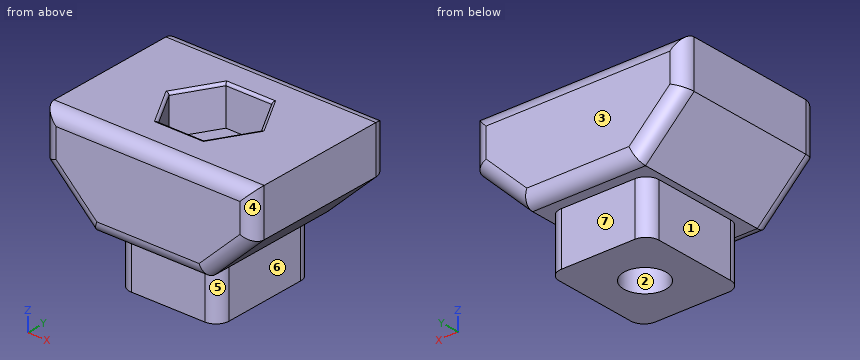
from build123d import *

# Parameters (mm, degrees)
BOSS_EXTRUDE1_DEPTH = 6
SKETCH2_W           = 7.6
SKETCH2_H           = 8.4
BOSS_EXTRUDE2_DEPTH = 4
FILLET1_R           = 1
SKETCH3_R           = 1.6
CUT_EXTRUDE1_DEPTH  = 12.2
FILLET2_R           = 1
CUT_EXTRUDE2_DEPTH  = 3
FILLET3_R           = 0.2


with BuildPart() as part:
    # Sketch1 → Boss-Extrude1 (new body, symmetric)
    with BuildSketch(Plane(origin=(0, 0, 0), x_dir=(1, 0, 0), z_dir=(0, 1, 0))):
        Polygon((-8, 0), (8, 0), (8, 3.6), (4.3, 7.2), (-4.3, 7.2), (-8, 3.6), align=None)
    extrude(amount=BOSS_EXTRUDE1_DEPTH, both=True)

    # Sketch2 → Boss-Extrude2 (add)
    with BuildSketch(Plane(origin=(0, 0, -7.2), x_dir=(-1, 0, 0), z_dir=(0, 0, -1))):
        Rectangle(SKETCH2_W, SKETCH2_H)
    extrude(amount=BOSS_EXTRUDE2_DEPTH)

    # Fillet1
    fillet1_edges = [part.edges().sort_by_distance(p)[0] for p in [
        (-6.15, 6, -5.4),
        (-8, 6, -1.8),
        (0, 6, 0),
        (8, 6, -1.8),
        (6.15, 6, -5.4),
        (8, -6, -1.8),
        (0, -6, 0),
        (-8, -6, -1.8),
        (-6.15, -6, -5.4),
        (0, -6, -7.2),
        (6.15, -6, -5.4),
        (0, 6, -7.2),
    ]]
    fillet(fillet1_edges, radius=FILLET1_R)

    # Sketch3 → Cut-Extrude1 (cut, through all)
    with BuildSketch(Plane(origin=(0, 0, -11.2), x_dir=(-1, 0, 0), z_dir=(0, 0, -1))):
        Circle(SKETCH3_R)
    extrude(amount=-CUT_EXTRUDE1_DEPTH, mode=Mode.SUBTRACT)

    # Fillet2
    fillet2_edges = [part.edges().sort_by_distance(p)[0] for p in [
        (-3.8, -4.2, -9.2),
        (-3.8, 4.2, -9.2),
        (3.8, 4.2, -9.2),
        (3.8, -4.2, -9.2),
    ]]
    fillet(fillet2_edges, radius=FILLET2_R)

    # Sketch4 → Cut-Extrude2 (cut)
    with BuildSketch(Plane.XY):
        Polygon((3.5, 0), (1.75, 3.031088913), (-1.75, 3.031088913), (-3.5, 0), (-1.75, -3.031088913), (1.75, -3.031088913), align=None)
    extrude(amount=-CUT_EXTRUDE2_DEPTH, mode=Mode.SUBTRACT)

    # Fillet3
    fillet3_edges = [part.edges().sort_by_distance(p)[0] for p in [
        (2.625, -1.515544457, 0),
        (2.625, 1.515544457, 0),
        (0, 3.031088913, 0),
        (-2.625, 1.515544457, 0),
        (-2.625, -1.515544457, 0),
        (0, -3.031088913, 0),
    ]]
    fillet(fillet3_edges, radius=FILLET3_R)


solid = part.part
Here's how the part is built. I have some questions about the finished solid (model axes, mm). Face numbers are marked on the shaded views. A direction names the side the tool comes from. Coordinates: 2 decimals unless noted, no trailing zeros. Order: outer loops, then holes, each group sorted by start corner. A loop starts at its lowest first (then second) coordinate and runs counter-clockwise, first axis right, second up.
Item 1: If we section it at C-C on y = 4.5: List the corners of the cut face in (x, z) for me, plus the area to 3 significant figures.
Result sheet:
outline: (-8, -3.6) - (-4.3, -7.2) - (4.3, -7.2) - (8, -3.6) - (8, 0) - (-8, 0) - close
area: 102 mm2
Item 2: For the marked faces 5, 6 and 7, which set-ups out of +Z, -Z, +X, -X, +Y, -Y let a thin tool reach every point of the face, with its end or its side?
Result sheet:
face 5: -Z, +X, -Y
face 6: -Z, +X, +Y, -Y
face 7: -Z, +X, -X, +Y
Item 3: For P1, Ø4.5, axis at x = -1, z = -10, coming from the -Y side; P2, Ø3, axis at x = 0, z = -8.5, coming from the +Y side; P3, Ø4.5, axis at y = -1, z = -9, coming from the -X side, each with a flat end and sliding along its axis, tell me the tip position at first contact or that it passes through.
Result sheet:
P1: stops at y = -4.2
P2: stops at y = 5.6
P3: stops at x = -4.76
Item 4: I need wall thicknesses on line 1 (Y direction, x = 0, z = -6.25); line 2 (Z direction, x = -2.25, y = -1.25); line 3 (Z direction, x = 3.5, y = -4.25). Which ranges of each line are inside material? Lowest first, please.
Result sheet:
line 1: y = -6 to -1.6, 1.6 to 6
line 2: z = -11.2 to -3
line 3: z = -7.2 to 0
Item 5: If we section it at A-A on z = -1.5: List the corners of the cut face in (x, y) for me, plus the area to 3 significant figures.
Result sheet:
outline: (-8, -5) arc R1 ccw to (-7, -6) - (7, -6) arc R1 ccw to (8, -5) - (8, 5) arc R1 ccw to (7, 6) - (-7, 6) arc R1 ccw to (-8, 5) - close; hole (-3.5, 0) - (-1.75, -3.03) - (1.75, -3.03) - (3.5, 0) - (1.75, 3.03) - (-1.75, 3.03) - close
area: 159 mm2
Item 6: If we mould it in two halves opening along X, with no side actions, what happens to the marked faces 1, 2, 3 and 4? For each: +X half, -X half, draft (parallel to the pull), parting line (faces both ways), or undercut.
Result sheet:
face 1: -X half
face 2: undercut
face 3: draft
face 4: +X half
Item 7: If we section it at D-D on z = -9.5: List the corners of the cut face in (x, y) for me, plus the area to 3 significant figures.
Result sheet:
outline: (-3.8, -3.2) arc R1 ccw to (-2.8, -4.2) - (2.8, -4.2) arc R1 ccw to (3.8, -3.2) - (3.8, 3.2) arc R1 ccw to (2.8, 4.2) - (-2.8, 4.2) arc R1 ccw to (-3.8, 3.2) - close; hole circle Ø3.2 at (0, 0)
area: 54.9 mm2
Item 8: If we section it at B-B on x = 0: List the corners of the cut face in (y, z) for me, plus the area to 3 significant figures.
Result sheet:
outline: (-6, -6.2) arc R1 ccw to (-5, -7.2) - (-4.2, -7.2) - (-4.2, -11.2) - (-1.6, -11.2) - (-1.6, -3) - (-3.03, -3) - (-3.03, -0.2) arc R0.2 ccw to (-3.23, 0) - (-5, 0) arc R1 ccw to (-6, -1) - close; (1.6, -11.2) - (4.2, -11.2) - (4.2, -7.2) - (5, -7.2) arc R1 ccw to (6, -6.2) - (6, -1) arc R1 ccw to (5, 0) - (3.23, 0) arc R0.2 ccw to (3.03, -0.2) - (3.03, -3) - (1.6, -3) - close
area: 74.7 mm2
